from build123d import *

# Parameters (mm, degrees)
F0_W     = 37.619051
F0_H     = 46.446688
F1_DEPTH = 25
F2_W     = 121.315539
F2_H     = 80.761321
F3_DEPTH = 5
F4_R     = 6.609922
F5_DEPTH = 25
F7_D     = 24


with BuildPart() as f1:
    # F0 (on Top) → F1 (new body)
    with BuildSketch(Plane.XY):
        with Locations((-18.809525, -23.223344)):
            Rectangle(F0_W, F0_H)
    extrude(amount=F1_DEPTH)

    # F2 (on face) → F3 (join)
    with BuildSketch(Plane.XY.offset(25)):
        with Locations((-20.51305, -22.998762)):
            Rectangle(F2_W, F2_H)
    extrude(amount=F3_DEPTH)

    # F4 (on face) → F5 (join)
    with BuildSketch(Plane.XY.offset(30)):
        with Locations((-39.504733, -40.390346)):
            Circle(F4_R)
    extrude(amount=F5_DEPTH)

    # F7 (through all)
    with Locations(Plane.XY.offset(30)):
        with Locations((19.895032, -50.992895)):
            Hole(F7_D / 2)


solid = f1.part
Could you check a few things on this model? Use its own coordinates, in mm. A direction names the side the tool comes from. Round coordinates to 2 decimals unless told otherwise and drop trailing zeros. Loops run counter-clockwise (first coordinate to the right, second up) from the corner with the lowest first, then second, coordinate; pieces in that order, holes last. Notation, with made-up numbers: (36, 43) - (82, 43) arc R21 cw to (82, 58) - close; hole circle Ø11 at (73, -7). An arc over 180 degrees is marked (long way). Write item = value, one per line.
1) Imagine slicing it at B-B (y = -12). Please give me the cut outline in (x, z).
Computed:
outline = (-81.17, 25) - (-37.62, 25) - (-37.62, 0) - (0, 0) - (0, 25) - (40.14, 25) - (40.14, 30) - (-81.17, 30) - close
2) On a 3-axis mill with a long thin cutter (end or side, diameter ignored), from which of +Z, -Z, +X, -X, +Y, -Y can I reach the whole of each face in a straight line? I mean faces 1 (the flat face through (-19, -46.447, 12)), 2 (the flat face through (-37.619, -24, 12)), 3 (the flat face through (0, -24, 12)). Say none if no direction works.
Computed:
face_1 = -Z, +X, -X, -Y
face_2 = -Z, -X, +Y, -Y
face_3 = -Z, +X, +Y, -Y
3) Imagine slicing it at C-C (x = -8). Please give me the cut outline in (y, z), and give its area (3 significant figures).
Computed:
outline = (-63.38, 25) - (-46.45, 25) - (-46.45, 0) - (0, 0) - (0, 25) - (17.38, 25) - (17.38, 30) - (-63.38, 30) - close
area = 1,560 mm2
4) I'm going to push flat-ended pins straight in: P1, Ø5, axis at x = -46, y = -27.5, coming from the -Z side; P2, Ø1.5, axis at x = -31.5, z = 38.5, coming from the -Y side; P3, Ø5, axis at y = -15.5, z = 6.5, coming from the -X side; P4, Ø20, axis at x = -10, z = 10.5, coming from the +Y side. Where does each tip first touch, or does it pass through?
Computed:
P1 = 25
P2 = through
P3 = -37.62
P4 = 0
5) Imagine slicing it at D-D (z = 15). Please give me the cut outline in (x, y).
Computed:
outline = (-37.62, -46.45) - (0, -46.45) - (0, 0) - (-37.62, 0) - close
6) Imagine slicing it at A-A (x = 16.5). Please give me the cut outline in (y, z), and give its area (3 significant figures).
Computed:
outline = (-63.38, 25) - (-62.5, 25) - (-62.5, 30) - (-63.38, 30) - close; (-39.48, 25) - (17.38, 25) - (17.38, 30) - (-39.48, 30) - close
area = 289 mm2
7) I need wall thicknesses on line 1 along X through (y, z) = (-20, 4); line 2 along Z through (x, y) = (-54, -9.5); line 3 along Z through (x, y) = (-17.5, -12). Which ranges of each line are inside material? Lowest first, please. Write a range as from..to.
Computed:
line_1 = -37.62..0
line_2 = 25..30
line_3 = 0..30
8) If we mould it in two halves opening along X, with no side actions, what happens to faces 4 (the cylindrical face through (29.42, -58.29, 27.47)), 5 (the flat face through (-48, -22, 25)), 6 (the cylindrical face through (-36.45, -46.25, 42.32))? For each: pulls with the +X half, pulls with the -X half, needs draft (parallel to the pull), parting line crosses it, or undercut.
Computed:
face_4 = undercut
face_5 = needs draft
face_6 = parting line crosses it
